Geometry: final body of the model. Coordinates: model frame, mm. A direction names the side the tool comes from. Round coordinates to 2 decimals unless told otherwise and drop trailing zeros. Loops run counter-clockwise (first coordinate to the right, second up) from the corner with the lowest first, then second, coordinate; pieces in that order, holes last. Notation, with made-up numbers: M 30.25,77.5 L 53.25,77.5 A9 cw 53.25,94.5 Z; hole C 76,-20.75 d2. An arc over 180 degrees is marked long. Write each question's results on one line, items separated by ' | '.
Autodesk Inventor part; units mm, degrees
ref_plane "YZ Plane" through (0, 0, 0) normal (1, 0, 0) x (0, 1, 0)
ref_plane "XZ Plane" through (0, 0, 0) normal (0, 1, 0) x (-1, 0, 0)
ref_plane "XY Plane" through (0, 0, 0) normal (0, 0, 1) x (1, 0, 0)
sketch "Sketch1" plane through (0, 0, 0) normal (0, 1, 0) x (-1, 0, 0)
  line L0 (-15, -15) -> (15, -15)
  line L1 (15, -15) -> (15, 15)
  line L2 (15, 15) -> (-15, 15)
  line L3 (-15, 15) -> (-15, -15)
  line L4 (-15, -15) -> (15, 15) construction
  line L5 (15, -15) -> (-15, 15) construction
  point P0 (0, 0)
  dimension "d0" = 30
  dimension "d1" = 30
extrude "Extrusion1" add sketch "Sketch1" along normal blind 2.5
sketch "Sketch2" plane through (0, 2.5, 0) normal (0, 1, 0) x (1, 0, 0)
  line L0 (15, -15) -> (15, 15)
  line L1 (15, -10) -> (-10, -10)
  line L2 (-10, -10) -> (-10, 10)
  line L3 (-10, 10) -> (15, 10)
  line L4 (15, 10) -> (15, -10)
  point P0 (0, 0)
  point P1 (15, 10)
  dimension "d4" = 20
  dimension "d5" = 10
  dimension "d6" = 25
extrude "Extrusion2" cut sketch "Sketch2" against normal through all
sketch "Sketch3" plane through (0, 2.5, 0) normal (0, 1, 0) x (1, 0, 0)
  line L0 (15, -10) -> (-10, -10)
  line L1 (-10, -10) -> (-10, 10)
  line L2 (-10, 10) -> (15, 10)
  line L3 (15, -10) -> (-10, -10)
  line L4 (-10, -10) -> (-10, -9)
  line L5 (-6.5, -9) -> (14, -9)
  line L6 (15, -10) -> (15, -10)
  line L7 (15, 10) -> (-10, 10)
  line L8 (-10, 10) -> (-10, 9)
  line L9 (-6.5, 9) -> (14, 9)
  line L10 (15, 10) -> (15, 10)
  line L11 (-10, -10) -> (-7.5, -10)
  line L12 (-7.5, -8) -> (-7.5, 8)
  line L13 (-7.5, 10) -> (-10, 10)
  line L14 (-10, 10) -> (-10, -10)
  arc A0 (15, -10) -> (14, -9) centre (14, -10) ccw
  arc A1 (-7.5, -8) -> (-6.5, -9) centre (-6.5, -8) ccw
  arc A2 (-6.5, 9) -> (-7.5, 8) centre (-6.5, 8) ccw
  arc A3 (14, 9) -> (15, 10) centre (14, 10) ccw
  point P0 (0, 0)
  point P1 (15, -9)
  point P2 (15, 9)
  point P3 (-7.5, -9)
  point P4 (-7.5, 9)
  dimension "d9" = 1
  dimension "d10" = 1
  dimension "d11" = 2.5
  dimension "d14" = 1
extrude "Extrusion3" add sketch "Sketch3" against normal blind 0.4
sketch "Sketch4" plane through (0, 2.5, 0) normal (0, 1, 0) x (1, 0, 0)
  point P0 (0, 0)
  point P1 (12.5, -12.5)
  point P2 (-12.5, -12.5)
  point P3 (-12.5, 12.5)
  point P4 (12.5, 12.5)
  point P5 (-12.5, 0)
  point P6 (0, -12.5)
  point P7 (0, 12.5)
  dimension "d15" = 25
  dimension "d16" = 25
  dimension "d17" = 12.5
  dimension "d18" = 12.5
hole "Hole1" at (12.5, 2.5, 12.5) at (-12.5, 2.5, 12.5) at (-12.5, 2.5, -12.5) at (12.5, 2.5, -12.5) at (0, 2.5, 12.5) at (0, 2.5, -12.5) direction (0, -1, 0) diameter 2.25 end through all counterbore diameter 3.5 counterbore depth 1.5
equation "\"d10\" = d9"
properties part number "Flex Circuit Clamp V1"
1. Section C-C (x = -12.5). Output: boundary loops of the cut face in (y, z) (3 decimals), then the cut area to 3 significant figures.
Answer key:
outline: M 0,-15 L 2.5,-15 L 2.5,-14.25 L 1,-14.25 L 1,-13.625 L 0,-13.625 Z; M 0,-11.375 L 1,-11.375 L 1,-10.75 L 2.5,-10.75 L 2.5,10.75 L 1,10.75 L 1,11.375 L 0,11.375 Z; M 0,13.625 L 1,13.625 L 1,14.25 L 2.5,14.25 L 2.5,15 L 0,15 Z | area: 60.0 mm²
2. Section D-D (y = 1.55). Output: boundary loops of the cut face in (x, z), then the cut area to 3 significant figures.
Answer key:
outline: M -15,-15 L 15,-15 L 15,-10 L -10,-10 L -10,10 L 15,10 L 15,15 L -15,15 Z; hole C -12.5,-12.5 d3.5; hole C -12.5,12.5 d3.5; hole C 0,-12.5 d3.5; hole C 0,12.5 d3.5; hole C 12.5,-12.5 d3.5; hole C 12.5,12.5 d3.5 | area: 342 mm²
3. Section B-B (x = -2.75). Output: boundary loops of the cut face in (y, z), then the cut area to 3 significant figures.
Answer key:
outline: M 0,-15 L 2.5,-15 L 2.5,-9 L 2.1,-9 L 2.1,-10 L 0,-10 Z; M 0,10 L 2.1,10 L 2.1,9 L 2.5,9 L 2.5,15 L 0,15 Z | area: 25.8 mm²
4. Ray query, probe 1 along Z at (x, y) = (-12.5, 1.95); probe 2 along X at (y, z) = (2.15, 12.5); probe 3 along Z at (x, y) = (0, 2.05). Return the intervals inside material, ascending.
Answer key:
probe 1: z = -15 to -14.25, -10.75 to 10.75, 14.25 to 15 | probe 2: x = -15 to -14.25, -10.75 to -1.75, 1.75 to 10.75, 14.25 to 15 | probe 3: z = -15 to -14.25, -10.75 to -10, 10 to 10.75, 14.25 to 15
5. Draft query along Z for faces 1 (the face through (11, 1.7, 13.4)), 2 (the face through (-15, 1, 0)), 3 (the face through (0, 1, 15)). Return one class per face: pulls with the +Z half, pulls with the -Z half, needs draft (parallel to the pull), parting line crosses it, or undercut.
Answer key:
face 1: undercut | face 2: needs draft | face 3: pulls with the +Z half
6. Access query for faces 4 (the face through (-8, 2.1, 0)), 5 (the face through (14.715, 2.303, 9.301)), 6 (the face through (14, 1, 12)). Directions: +Z, -Z, +X, -X, +Y, -Y. A direction counts if a zero-diameter tool reaches every point of the face in a straight line with its end or side. Return the directions, or none.
Answer key:
face 4: +X, -Y | face 5: +X, +Y, -Y | face 6: +Y
7. Pin query (flat end, axial travel): P1, Ø2, axis at x = 12.5, z = 12.5, coming from the +Y side; P2, Ø1.8, axis at x = -12.5, z = 13, coming from the +Y side; P3, Ø1, axis at y = 0.5, z = -2, coming from the +X side. Return the tip coordinate at first contact, or that it passes through.
Answer key:
P1: passes through | P2: stops at y = 1 | P3: stops at x = -10
8. Section A-A (z = 12.5). Output: boundary loops of the cut face in (x, y) (3 decimals), then the cut area to 3 significant figures.
Answer key:
outline: M -15,0 L -13.625,0 L -13.625,1 L -14.25,1 L -14.25,2.5 L -15,2.5 Z; M -11.375,0 L -1.125,0 L -1.125,1 L -1.75,1 L -1.75,2.5 L -10.75,2.5 L -10.75,1 L -11.375,1 Z; M 1.125,0 L 11.375,0 L 11.375,1 L 10.75,1 L 10.75,2.5 L 1.75,2.5 L 1.75,1 L 1.125,1 Z; M 13.625,0 L 15,0 L 15,2.5 L 14.25,2.5 L 14.25,1 L 13.625,1 Z | area: 52.5 mm²
